The listing builds one solid part. Answer for the finished solid, in the listing's coordinates (mm). Round coordinates to 2 decimals unless told otherwise and drop trailing zeros. Write each loop counter-clockwise with the first axis right and the second up, starting at its lowest first coordinate (ties: lowest second). Pieces come first, ordered by that corner, then holes. Notation, with made-up numbers: (45.25, 61) - (87.25, 61) arc R29 cw to (87.25, 85) - close; hole circle Ø7 at (1.25, 43). An arc over 180 degrees is marked (long way). Answer in a Markdown table with one row per item.
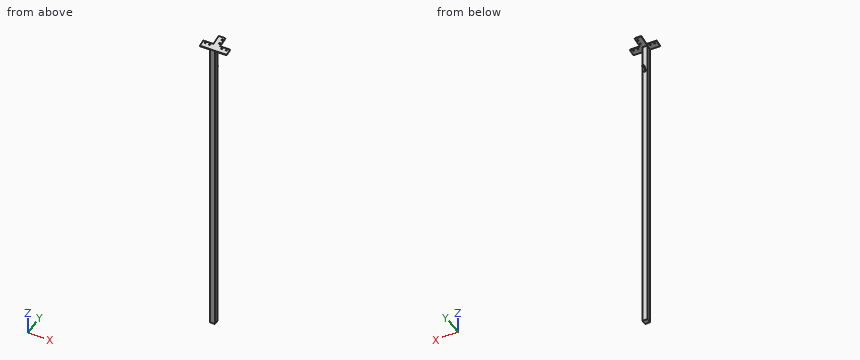
from build123d import *

# Parameters (mm, degrees)
F0_W          = 45
F0_H          = 45
F1_DEPTH      = 2795
F3_W          = 45
F3_H          = 60
F3_W_2        = 90
F4_DEPTH      = 5
F6_DEPTH      = 45
F8_W          = 2.7798460424
F8_H          = 5.7082939148
F9_DEPTH      = 150
F9_DEPTH_BACK = 90
F10_R         = 6
F11_DEPTH     = 5
F15_DEPTH     = 30


with BuildPart() as f1:
    # F0 (on Top) → F1 (new body)
    with BuildSketch(Plane.XY):
        Rectangle(F0_W, F0_H)
    extrude(amount=F1_DEPTH)


with BuildPart() as f4:
    # F3 (on face) → F4 (new body)
    with BuildSketch(Plane(origin=(0, -524.3318959349, 2697.453760933), x_dir=(1, 0, 0), z_dir=(0, -0.1908089954, 0.9816271834))):
        with Locations((0, 541.2245304499)):
            Rectangle(F3_W, F3_H)
        with Locations((-67.5, 541.2245304499)):
            Rectangle(F3_W_2, F3_H)
        Polygon((22.5, 571.2245304499), (22.5, 511.2245304499), (37.5, 511.2245304499), (37.5, 571.2245304499), (37.5, 661.2245304499), (-22.5, 661.2245304499), (-22.5, 571.2245304499), align=None)
        with Locations((82.5, 541.2245304499)):
            Rectangle(F3_W_2, F3_H)
    extrude(amount=F4_DEPTH)


with BuildPart() as f6:
    # F5 (on face) → F6 (new body)
    with BuildSketch(Plane.YZ.offset(22.5)):
        Polygon((-22.5, 2795), (22.5, 2795), (22.5, 2803.7471139112), align=None)
    extrude(amount=-F6_DEPTH)


with BuildPart() as f1_1:
    add(f1.part)

    # F7: union F6, F4
    add(f6.part)
    add(f4.part)

    # F8 (on face) → F9 (cut, two sides)
    with BuildSketch(Plane(origin=(-22.5, 0, 0), x_dir=(0, -1, 0), z_dir=(-1, 0, 0))) as f9_sk:
        with Locations((23.8899230212, 2797.8541469574)):
            Rectangle(F8_W, F8_H)
    extrude(amount=-F9_DEPTH, mode=Mode.SUBTRACT)
    extrude(f9_sk.sketch, amount=F9_DEPTH_BACK, mode=Mode.SUBTRACT)

    # F10 (on face) → F11 (cut, through all)
    with BuildSketch(Plane(origin=(0, -525.2859409117, 2702.3618968503), x_dir=(1, 0, 0), z_dir=(0, -0.1908089954, 0.9816271834))):
        with BuildLine():
            ThreePointArc((108.5, 556.2245304499), (106.7426406871, 560.467171137), (102.5, 562.2245304499))
            Line((102.5, 562.2245304499), (102.5, 556.2245304499))
            Line((102.5, 556.2245304499), (96.5, 556.2245304499))
            ThreePointArc((96.5, 556.2245304499), (102.5, 550.2245304499), (108.5, 556.2245304499))
        make_face()
        with Locations((62.5, 556.2245304499)):
            Circle(F10_R)
        with BuildLine():
            Line((102.5, 556.2245304499), (102.5, 562.2245304499))
            ThreePointArc((102.5, 562.2245304499), (98.2573593129, 560.467171137), (96.5, 556.2245304499))
            Line((96.5, 556.2245304499), (102.5, 556.2245304499))
        make_face()
        with BuildLine():
            ThreePointArc((22.5, 630.2245304499), (26.7426406871, 631.9818897628), (28.5, 636.2245304499))
            Line((28.5, 636.2245304499), (22.5, 636.2245304499))
            Line((22.5, 636.2245304499), (22.5, 630.2245304499))
        make_face()
        with BuildLine():
            Line((22.5, 636.2245304499), (28.5, 636.2245304499))
            ThreePointArc((28.5, 636.2245304499), (18.2573593129, 640.467171137), (22.5, 630.2245304499))
            Line((22.5, 630.2245304499), (22.5, 636.2245304499))
        make_face()
        with BuildLine():
            ThreePointArc((28.5, 596.2245304499), (26.7426406871, 600.467171137), (22.5, 602.2245304499))
            ThreePointArc((22.5, 602.2245304499), (18.2573593129, 591.9818897628), (28.5, 596.2245304499))
        make_face()
        with Locations((-47.5, 556.2245304499)):
            Circle(F10_R)
        with Locations((-87.5, 556.2245304499)):
            Circle(F10_R)
    extrude(amount=-F11_DEPTH, mode=Mode.SUBTRACT)

    # F14 (on offset) → F15 (join)
    with BuildSketch(Plane.XY.offset(2545)):
        with BuildLine():
            Line((0, 27.5), (5, 27.5))
            ThreePointArc((5, 27.5), (0, 32.5), (-5, 27.5))
            Line((-5, 27.5), (0, 27.5))
        make_face()
        with BuildLine():
            Line((5, 22.5), (5, 27.5))
            ThreePointArc((5, 27.5), (3.5355339059, 23.9644660941), (0, 22.5))
            Line((0, 22.5), (5, 22.5))
        make_face()
        with BuildLine():
            ThreePointArc((0, 22.5), (3.5355339059, 23.9644660941), (5, 27.5))
            Line((5, 27.5), (0, 27.5))
            Line((0, 27.5), (0, 22.5))
        make_face()
        with BuildLine():
            Line((0, 27.5), (-5, 27.5))
            ThreePointArc((-5, 27.5), (-3.5355339059, 23.9644660941), (0, 22.5))
            Line((0, 22.5), (0, 27.5))
        make_face()
        with BuildLine():
            ThreePointArc((0, 22.5), (-3.5355339059, 23.9644660941), (-5, 27.5))
            Line((-5, 27.5), (-5, 22.5))
            Line((-5, 22.5), (0, 22.5))
        make_face()
    extrude(amount=F15_DEPTH)

    # F17: sweep along a path in F13
    with BuildLine(Plane.YZ) as f17_path:
        ThreePointArc((57.5, 2575), (42.5, 2590), (27.5, 2575))
    # F16 (on face) → F17 (sweep)
    with BuildSketch(Plane.XY.offset(2575)):
        with BuildLine():
            ThreePointArc((0, 22.5), (3.5355339059, 23.9644660941), (5, 27.5))
            ThreePointArc((5, 27.5), (0, 32.5), (-5, 27.5))
            ThreePointArc((-5, 27.5), (-3.5355339059, 23.9644660941), (0, 22.5))
        make_face()
    sweep(path=f17_path.line)


solid = f1_1.part
(1) Flat-ended cylindrical pins translate along their axes: pin 1 (11 mm diameter, centred on y = 82.5, z = 2820, fed in from +X); pin 2 (5 mm diameter, centred on x = 0, y = 59, fed in from -Z); pin 3 (5.5 mm diameter, centred on x = -2, y = 24.5, fed in from +Z). Find the tip coordinate at first contact, or state that the pin passes through.
Checked values:
| item | result |
|---|---|
| pin 1 | stops at x = 37.5 |
| pin 2 | stops at z = 2575 |
| pin 3 | stops at z = 2809.76 |
(2) Section A-A (z = 1357.5) is taken. Give the vertices of the cut face in (x, y).
Checked values:
| item | result |
|---|---|
| outline | (-22.5, -22.5) - (22.5, -22.5) - (22.5, 22.5) - (-22.5, 22.5) - close |
(3) Find the intervals of material crossed by line 1 (X direction, y = -7, z = 1140); line 2 (Z direction, x = 73.5, y = 9.5), in increasing order.
Checked values:
| item | result |
|---|---|
| line 1 | x = -22.5 to 22.5 |
| line 2 | z = 2801.22 to 2806.31 |
